Check sheet for the modelled part. Datum: model origin and axes. Units: mm. A direction names the side the tool comes from. Give positions to 0.01 mm unless a question says otherwise; leave off trailing zeros. Order: outer loops, then holes, each group sorted by start corner. A loop starts at its lowest first (then second) coordinate and runs counter-clockwise, first axis right, second up.
```python
from build123d import *

# Parameters (mm, degrees)
SKETCH1_R           = 25
BOSS_EXTRUDE1_DEPTH = 20
BOSS_EXTRUDE2_DEPTH = 15
SKETCH3_R           = 2
BOSS_EXTRUDE3_DEPTH = 1
CUT_EXTRUDE1_DEPTH  = 2


with BuildPart() as part:
    # Sketch1 → Boss-Extrude1 (new body)
    with BuildSketch(Plane(origin=(0, 0, 0), x_dir=(0, 0, -1), z_dir=(1, 0, 0))):
        Circle(SKETCH1_R)
    extrude(amount=BOSS_EXTRUDE1_DEPTH)

    # Sketch2 → Boss-Extrude2 (add)
    with BuildSketch(Plane(origin=(20, 0, 0), x_dir=(0, 0, -1), z_dir=(1, 0, 0))):
        with BuildLine():
            Line((-2.449489743, 12.5), (2.449489743, 12.5))
            ThreePointArc((2.449489743, 12.5), (0, 18.5), (-2.449489743, 12.5))
        make_face()
    extrude(amount=BOSS_EXTRUDE2_DEPTH)

    # Sketch3 → Boss-Extrude3 (add)
    with BuildSketch(Plane(origin=(20, 0, 0), x_dir=(0, 0, -1), z_dir=(1, 0, 0))):
        with BuildLine():
            Line((-31.854729385, 3), (-30.392824551, -10))
            Line((-30.392824551, -10), (-22.912878475, -10))
            ThreePointArc((-22.912878475, -10), (-24.735426905, -3.62748616), (-24.819347292, 3))
            Line((-24.819347292, 3), (-31.854729385, 3))
        make_face()
        with Locations((-28.497841918, 0)):
            Circle(SKETCH3_R, mode=Mode.SUBTRACT)
        with Locations((-27.624753284, -7)):
            Circle(SKETCH3_R, mode=Mode.SUBTRACT)
        with BuildLine():
            Line((31.854729385, 3), (30.392824551, -10))
            Line((30.392824551, -10), (22.912878475, -10))
            ThreePointArc((22.912878475, -10), (24.735426905, -3.62748616), (24.819347292, 3))
            Line((24.819347292, 3), (31.854729385, 3))
        make_face()
        with Locations((27.624753284, -7)):
            Circle(SKETCH3_R, mode=Mode.SUBTRACT)
        with Locations((28.497841918, 0)):
            Circle(SKETCH3_R, mode=Mode.SUBTRACT)
    extrude(amount=-BOSS_EXTRUDE3_DEPTH)

    # Sketch4 → Cut-Extrude1 (cut)
    with BuildSketch(Plane(origin=(35, 0, 0), x_dir=(0, 0, -1), z_dir=(1, 0, 0))):
        with BuildLine():
            Line((0, 15), (3.5, 15))
            ThreePointArc((3.5, 15), (-2.474873734, 12.525126266), (0, 18.5))
            Line((0, 18.5), (0, 15))
        make_face()
    extrude(amount=-CUT_EXTRUDE1_DEPTH, mode=Mode.SUBTRACT)


solid = part.part
```
Q1. Sectioned sample at C-C, the plane y = 9. Record the cut outline in (x, z), plus the area to 3 significant figures.
Q2. Tool access check on faces 1 (the flat face through (26, 12.5, 0)), 2 (the cylindrical face through (9.86, 7.509, -23.846)), 3 (the cylindrical face through (27.4, 18.5, -0.1)). Record the directions out of +Z, -Z, +X, -X, +Y, -Y that give a thin tool (end or side, any length) a straight path to the whole face; none if there is none.
Q3. Sectioned sample at A-A, the plane y = 0. Record the cut outline in (x, z).
Q4. Go/stop test with flat-tipped pins: P1, Ø1.5, axis at x = 6.5, z = 14.5, coming from the +Y side; P2, Ø4, axis at x = 24, z = 0, coming from the -Y side; P3, Ø0.6, axis at x = 34.5, y = 17, coming from the +Z side. Record where each tip stops, or that it passes through.
Q5. Sectioned sample at B-B, the plane z = 12. Record the cut outline in (x, y), plus the area to 3 significant figures.
Q6. Material ranges on line 1 (X direction, y = 10, z = 14.5); line 2 (Y direction, x = 14, z = -10); line 3 (Z direction, x = 15.5, y = 3.5), recorded low to high.
Q7. Draft check along Y on faces 4 (the flat face through (34, 17, 0)), 5 (the flat face through (34, 15, -2)), 6 (the cylindrical face through (19.51, 0.6, 26.59)), 7 (the cylindrical face through (19.507, -6.399, -29.532)). Enter one of: pulls with the +Y half, pulls with the -Y half, needs draft (parallel to the pull), parting line crosses it, or undercut.
Filled in:
1. outline: (0, -23.32) - (20, -23.32) - (20, 23.32) - (0, 23.32) - close
1. area: 933 mm2
2. face 1: +Z, -Z, +X, -Y
2. face 2: -X
2. face 3: +X
3. outline: (0, -25) - (19, -25) - (19, -26.5) - (20, -26.5) - (20, 26.5) - (19, 26.5) - (19, 25) - (0, 25) - close; (19, -31.52) - (20, -31.52) - (20, -30.5) - (19, -30.5) - close; (19, 30.5) - (20, 30.5) - (20, 31.52) - (19, 31.52) - close
4. P1: stops at y = 20.88
4. P2: stops at y = 12.5
4. P3: stops at z = 0
5. outline: (0, -21.93) - (20, -21.93) - (20, 21.93) - (0, 21.93) - close
5. area: 877 mm2
6. line 1: x = 0 to 20
6. line 2: y = -22.91 to 22.91
6. line 3: z = -24.75 to 24.75
7. face 4: needs draft
7. face 5: pulls with the -Y half
7. face 6: undercut
7. face 7: undercut
